Work out the finished part from the listing and answer in its coordinate system (mm). Face numbers are marked on the shaded views. A direction names the side the tool comes from. Coordinates: 2 decimals unless noted, no trailing zeros. Order: outer loops, then holes, each group sorted by start corner. A loop starts at its lowest first (then second) coordinate and runs counter-clockwise, first axis right, second up.
1. The part is cut by section A-A, the plane x = 40.75. Give the vertices of the cut face in (y, z), then the cut area to 3 significant figures.
2. The part is cut by section D-D, the plane z = -7. Give the vertices of the cut face in (x, y).
3. Flat-ended cylindrical pins translate along their axes: pin 1 Ø0.5 at (x, z) = (42, -13) entering from +Y; pin 2 Ø0.7 at (x, z) = (39, 0) entering from -Y; pin 3 Ø5 at (y, z) = (17.5, -11.5) entering from -X. Find the tip coordinate at first contact, or state that the pin passes through.
4. The part is cut by section B-B, the plane z = -12. Give the vertices of the cut face in (x, y), then the cut area to 3 significant figures.
5. A tool of negligible diameter and unlimited length cuts with its end or side. For the marked faces 1 and 2, from which of +Z, -Z, +X, -X, +Y, -Y can it reach the whole face along a straight path? Write none if from no direction.
6. Determine the mould class of the marked faces 3, 4, 5 and 6 for opening direction Z: +Z half, -Z half, draft (parallel to the pull), parting line (faces both ways), or undercut.
7. Find the intervals of material crossed by probe 1 along Z at (x, y) = (36, 11.5); probe 2 along Z at (x, y) = (22.25, 7.5); probe 3 along Y at (x, z) = (42.5, -4.5), in increasing order.
8. The part is cut by section C-C, the plane y = 6. Give the vertices of the cut face in (x, z).
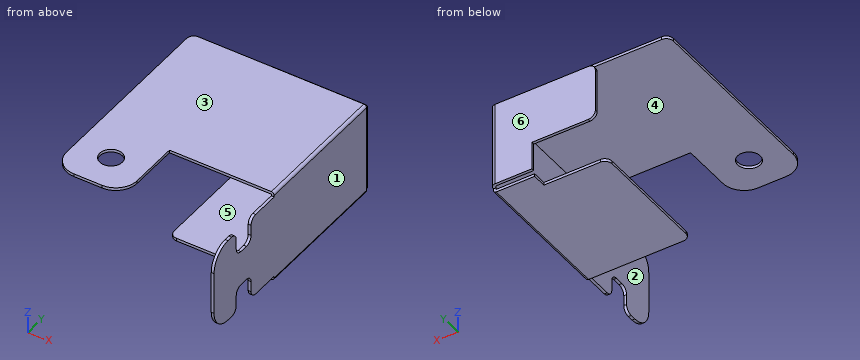
```python
from build123d import *

# Parameters (mm, degrees)
SKETCH1_R                   = 1.6
BASE_FLANGE1_DEPTH          = 0.4
SKETCHED_START              = 45.702497433
SKETCHED_BEND8_DEPTH        = 12
SKETCHED_BEND8_2_DEPTH      = 8
SKETCHED_START_2            = 53.702497433
SKETCHED_BEND8_3_DEPTH      = 4
SKETCHED_START_3            = -4.042672779
SKETCHED_BEND12_DEPTH       = 33.707300919
SKETCHED_START_4            = 8.957327221
SKETCHED_BEND12_2_DEPTH     = 18
SKETCHED_START_5            = 3.957327221
SKETCHED_BEND12_3_OUTLINE_W = 0.4
SKETCHED_BEND12_3_OUTLINE_H = 12
SKETCHED_BEND12_3_DEPTH     = 25.007300919
SKETCHED_BEND12_4_OUTLINE_W = 0.4
SKETCHED_BEND12_4_OUTLINE_H = 12
SKETCHED_BEND12_4_DEPTH     = 4.8
SKETCHED_START_6            = 0.757327221
SKETCHED_BEND12_5_OUTLINE_W = 0.4
SKETCHED_BEND12_5_OUTLINE_H = 5
SKETCHED_BEND12_5_DEPTH     = 3.2
SKETCHED_START_7            = 26.957327221
SKETCHED_BEND12_6_DEPTH     = 2
SKETCHED_START_8            = -8.643134969
SKETCHED_BEND12_7_DEPTH     = 8
SKETCHED_START_9            = -12.643134969
SKETCHED_BEND12_8_DEPTH     = 4
FILLET1_R                   = 3
FILLET2_R                   = 1
FILLET3_R                   = 1


with BuildPart() as part:
    # Base-Flange1: sheet metal written as solids
    # Sketch1 → Base-Flange1 (new body)
    with BuildSketch(Plane.XY):
        Polygon((30.702497433, -1.042672779), (30.702497433, 8.957327221), (45.702497433, 8.957327221), (45.702497433, 3.957327221), (49.202497433, 3.957327221), (49.202497433, 0.757327221), (45.702497433, 0.757327221), (45.702497433, -4.042672779), (57.702497433, -4.042672779), (57.702497433, 0.757327221), (54.202497433, 0.757327221), (54.202497433, 3.957327221), (57.702497433, 3.957327221), (57.702497433, 8.957327221), (72.702497433, 8.957327221), (72.702497433, 26.957327221), (63.702497433, 26.957327221), (63.702497433, 28.957327221), (57.702497433, 28.957327221), (57.702497433, 34.957327221), (53.702497433, 34.957327221), (53.702497433, 43.957327221), (45.702497433, 43.957327221), (45.702497433, 28.957327221), (20.702497433, 28.957327221), (20.702497433, -1.042672779), align=None)
        with Locations((25.702497433, 3.957327221)):
            Circle(SKETCH1_R, mode=Mode.SUBTRACT)
    extrude(amount=-BASE_FLANGE1_DEPTH)

    # Sketched Bend8: read off the stored shape, not the designer's step
    # Sketched Bend8 outline → Sketched Bend8 (cut)
    with BuildSketch(Plane.YZ.offset(SKETCHED_START)):
        with BuildLine():
            ThreePointArc((28.96462814, 0), (29.338793878, -0.108392022), (29.597083672, -0.4))
            Line((29.597083672, -0.4), (43.957327221, -0.4))
            Line((43.957327221, -0.4), (43.957327221, 0))
            Line((43.957327221, 0), (28.96462814, 0))
        make_face()
    extrude(amount=SKETCHED_BEND8_DEPTH, mode=Mode.SUBTRACT)

    # Sketched Bend8 2 outline → Sketched Bend8 2 (add)
    with BuildSketch(Plane.YZ.offset(SKETCHED_START)):
        with BuildLine():
            Line((29.26462814, -14.907300918), (29.66462814, -14.907300918))
            Line((29.66462814, -14.907300918), (29.66462814, -0.7))
            ThreePointArc((29.66462814, -0.7), (29.647533284, -0.546245118), (29.597083672, -0.4))
            Line((29.597083672, -0.4), (28.96462814, -0.4))
            ThreePointArc((28.96462814, -0.4), (29.176760174, -0.487867966), (29.26462814, -0.7))
            Line((29.26462814, -0.7), (29.26462814, -14.907300918))
        make_face()
    extrude(amount=SKETCHED_BEND8_2_DEPTH)

    # Sketched Bend8 3 outline → Sketched Bend8 3 (add)
    with BuildSketch(Plane.YZ.offset(SKETCHED_START_2)):
        with BuildLine():
            Line((29.26462814, -0.7), (29.26462814, -5.907300918))
            Line((29.26462814, -5.907300918), (29.66462814, -5.907300918))
            Line((29.66462814, -5.907300918), (29.66462814, -0.7))
            ThreePointArc((29.66462814, -0.7), (29.647533284, -0.546245118), (29.597083672, -0.4))
            Line((29.597083672, -0.4), (28.96462814, -0.4))
            ThreePointArc((28.96462814, -0.4), (29.176760174, -0.487867966), (29.26462814, -0.7))
        make_face()
    extrude(amount=SKETCHED_BEND8_3_DEPTH)

    # Sketched Bend12: read off the stored shape, not the designer's step
    # Sketched Bend12 outline → Sketched Bend12 (cut)
    with BuildSketch(Plane(origin=(0, 0, 0), x_dir=(1, 0, 0), z_dir=(0, 1, 0)).offset(SKETCHED_START_3)):
        with BuildLine():
            Line((45.702497433, 0.4), (45.545631155, 0.4))
            ThreePointArc((45.545631155, 0.4), (45.427828447, 0.117096847), (45.144632402, 0))
            Line((45.144632402, 0), (72.702497433, 0))
            Line((72.702497433, 0), (72.702497433, 0.4))
            Line((72.702497433, 0.4), (57.702497433, 0.4))
            Line((57.702497433, 0.4), (57.702497433, 5.907300918))
            Line((57.702497433, 5.907300918), (53.702497433, 5.907300918))
            Line((53.702497433, 5.907300918), (53.702497433, 14.907300918))
            Line((53.702497433, 14.907300918), (45.702497433, 14.907300918))
            Line((45.702497433, 14.907300918), (45.702497433, 0.4))
        make_face()
    extrude(amount=SKETCHED_BEND12_DEPTH, mode=Mode.SUBTRACT)

    # Sketched Bend12 2 outline → Sketched Bend12 2 (add)
    with BuildSketch(Plane(origin=(0, 0, 0), x_dir=(1, 0, 0), z_dir=(0, 1, 0)).offset(SKETCHED_START_4)):
        with BuildLine():
            ThreePointArc((45.145632402, 0.401), (45.145339509, 0.400292893), (45.144632402, 0.4))
            Line((45.144632402, 0.4), (45.545631155, 0.4))
            ThreePointArc((45.545631155, 0.4), (45.54563209, 0.4005), (45.545632402, 0.401))
            Line((45.545632402, 0.401), (45.545632402, 12.885269938))
            ThreePointArc((45.545632402, 12.885269938), (45.428182222, 13.168819758), (45.144632402, 13.286269938))
            Line((45.144632402, 13.286269938), (30.702497433, 13.286269938))
            Line((30.702497433, 13.286269938), (30.702497433, 12.886269938))
            Line((30.702497433, 12.886269938), (45.144632402, 12.886269938))
            ThreePointArc((45.144632402, 12.886269938), (45.145339509, 12.885977045), (45.145632402, 12.885269938))
            Line((45.145632402, 12.885269938), (45.145632402, 0.401))
        make_face()
    extrude(amount=SKETCHED_BEND12_2_DEPTH)

    # Sketched Bend12 3 outline → Sketched Bend12 3 (add)
    with BuildSketch(Plane(origin=(0, 0, 0), x_dir=(1, 0, 0), z_dir=(0, 1, 0)).offset(SKETCHED_START_5)):
        with Locations((45.345632402, 6.643134969)):
            Rectangle(SKETCHED_BEND12_3_OUTLINE_W, SKETCHED_BEND12_3_OUTLINE_H)
    extrude(amount=SKETCHED_BEND12_3_DEPTH)



with BuildPart() as body_2:
    # Sketched Bend12 4 outline → Sketched Bend12 4 (new body)
    with BuildSketch(Plane(origin=(0, 0, 0), x_dir=(1, 0, 0), z_dir=(0, 1, 0)).offset(SKETCHED_START_3)):
        with Locations((45.345632402, 6.643134969)):
            Rectangle(SKETCHED_BEND12_4_OUTLINE_W, SKETCHED_BEND12_4_OUTLINE_H)
    extrude(amount=SKETCHED_BEND12_4_DEPTH)


with BuildPart() as part_1:
    add(part.part)

    add(body_2.part)  # Sketched Bend12 5 merges body 2
    # Sketched Bend12 5 outline → Sketched Bend12 5 (add)
    with BuildSketch(Plane(origin=(0, 0, 0), x_dir=(1, 0, 0), z_dir=(0, 1, 0)).offset(SKETCHED_START_6)):
        with Locations((45.345632402, 6.643134969)):
            Rectangle(SKETCHED_BEND12_5_OUTLINE_W, SKETCHED_BEND12_5_OUTLINE_H)
    extrude(amount=SKETCHED_BEND12_5_DEPTH)

    # Sketched Bend12 6 outline → Sketched Bend12 6 (add)
    with BuildSketch(Plane(origin=(0, 0, 0), x_dir=(1, 0, 0), z_dir=(0, 1, 0)).offset(SKETCHED_START_7)):
        with BuildLine():
            Line((45.145632402, 0.643134969), (45.145632402, 0.401))
            ThreePointArc((45.145632402, 0.401), (45.145339509, 0.400292893), (45.144632402, 0.4))
            Line((45.144632402, 0.4), (45.545631155, 0.4))
            ThreePointArc((45.545631155, 0.4), (45.54563209, 0.4005), (45.545632402, 0.401))
            Line((45.545632402, 0.401), (45.545632402, 0.643134969))
            Line((45.545632402, 0.643134969), (45.145632402, 0.643134969))
        make_face()
        with BuildLine():
            Line((45.145632402, 12.885269938), (45.145632402, 12.643134969))
            Line((45.145632402, 12.643134969), (45.545632402, 12.643134969))
            Line((45.545632402, 12.643134969), (45.545632402, 12.885269938))
            ThreePointArc((45.545632402, 12.885269938), (45.428182222, 13.168819758), (45.144632402, 13.286269938))
            Line((45.144632402, 13.286269938), (39.702497433, 13.286269938))
            Line((39.702497433, 13.286269938), (39.702497433, 12.886269938))
            Line((39.702497433, 12.886269938), (45.144632402, 12.886269938))
            ThreePointArc((45.144632402, 12.886269938), (45.145339509, 12.885977045), (45.145632402, 12.885269938))
        make_face()
    extrude(amount=SKETCHED_BEND12_6_DEPTH)

    # Sketched Bend12 7 outline → Sketched Bend12 7 (add)
    with BuildSketch(Plane.XY.offset(SKETCHED_START_8)):
        with BuildLine():
            ThreePointArc((44.845632402, 29.26462814), (45.057764437, 29.176760175), (45.145632402, 28.96462814))
            Line((45.145632402, 28.96462814), (45.545632402, 28.96462814))
            ThreePointArc((45.545632402, 28.96462814), (45.340607148, 29.459602887), (44.845632402, 29.66462814))
            Line((44.845632402, 29.66462814), (30.638331484, 29.66462814))
            Line((30.638331484, 29.66462814), (30.638331484, 29.26462814))
            Line((30.638331484, 29.26462814), (44.845632402, 29.26462814))
        make_face()
    extrude(amount=SKETCHED_BEND12_7_DEPTH)

    # Sketched Bend12 8 outline → Sketched Bend12 8 (add)
    with BuildSketch(Plane.XY.offset(SKETCHED_START_9)):
        with BuildLine():
            Line((39.638331484, 29.26462814), (44.845632402, 29.26462814))
            ThreePointArc((44.845632402, 29.26462814), (45.057764437, 29.176760175), (45.145632402, 28.96462814))
            Line((45.145632402, 28.96462814), (45.545632402, 28.96462814))
            ThreePointArc((45.545632402, 28.96462814), (45.340607148, 29.459602887), (44.845632402, 29.66462814))
            Line((44.845632402, 29.66462814), (39.638331484, 29.66462814))
            Line((39.638331484, 29.66462814), (39.638331484, 29.26462814))
        make_face()
    extrude(amount=SKETCHED_BEND12_8_DEPTH)

    # Fillet1
    fillet1_edges = [part_1.edges().sort_by_distance(p)[0] for p in [
        (45.345632402, -4.042672779, -0.643134969),
        (45.345632402, -4.042672779, -12.643134969),
        (20.702497433, -1.042672779, -0.2),
        (30.702497433, -1.042672779, -0.2),
    ]]
    fillet(fillet1_edges, radius=FILLET1_R)

    # Fillet2
    fillet2_edges = [part_1.edges().sort_by_distance(p)[0] for p in [
        (20.702497433, 28.957327221, -0.2),
        (30.702497433, 26.957327221, -13.086269938),
        (30.702497433, 8.957327221, -13.086269938),
        (30.638331484, 29.46462814, -0.643134969),
        (30.638331484, 29.46462814, -8.643134969),
    ]]
    fillet(fillet2_edges, radius=FILLET2_R)

    # Fillet3
    fillet3_edges = [part_1.edges().sort_by_distance(p)[0] for p in [
        (45.345632402, 3.957327221, -0.643134969),
        (45.345632402, 3.957327221, -4.143134969),
        (45.345632402, 0.757327221, -4.143134969),
        (45.345632402, 0.757327221, -0.643134969),
        (45.345632402, 0.757327221, -12.643134969),
        (45.345632402, 0.757327221, -9.143134969),
        (45.345632402, 3.957327221, -9.143134969),
        (45.345632402, 3.957327221, -12.643134969),
    ]]
    fillet(fillet3_edges, radius=FILLET3_R)


solid = part_1.part
```
Geometry says:
1. outline: (8.96, -13.29) - (28.96, -13.29) - (28.96, -12.89) - (8.96, -12.89) - close; (8.96, -0.4) - (28.96, -0.4) - (28.96, 0) - (8.96, 0) - close; (29.26, -12.64) - (29.66, -12.64) - (29.66, -0.64) - (29.26, -0.64) - close
1. area: 20.8 mm2
2. outline: (30.64, 29.26) - (44.85, 29.26) arc R0.3 cw to (45.15, 28.96) - (45.15, -4.04) - (45.55, -4.04) - (45.55, 28.96) arc R0.7 ccw to (44.85, 29.66) - (30.64, 29.66) - close
3. pin 1: stops at y = 28.96
3. pin 2: stops at y = 8.96
3. pin 3: stops at x = 30.7
4. outline: (39.64, 29.26) - (44.85, 29.26) arc R0.3 cw to (45.15, 28.96) - (45.15, 4.02) - (45.55, 4.02) - (45.55, 28.96) arc R0.7 ccw to (44.85, 29.66) - (39.64, 29.66) - close; (45.15, -2.9) - (45.55, -2.9) - (45.55, 0.69) - (45.15, 0.69) - close
4. area: 13.8 mm2
5. face 1: +Z, -Z, +X, +Y, -Y
5. face 2: -X, -Y
6. face 3: +Z half
6. face 4: undercut
6. face 5: undercut
6. face 6: draft
7. probe 1: z = -13.29 to -12.89, -0.4 to 0
7. probe 2: z = -0.4 to 0
7. probe 3: y = 29.26 to 29.66
8. outline: (20.7, -0.4) - (30.7, -0.4) - (30.7, 0) - (20.7, 0) - close; (45.15, -12.64) - (45.55, -12.64) - (45.55, -0.64) - (45.15, -0.64) - close
